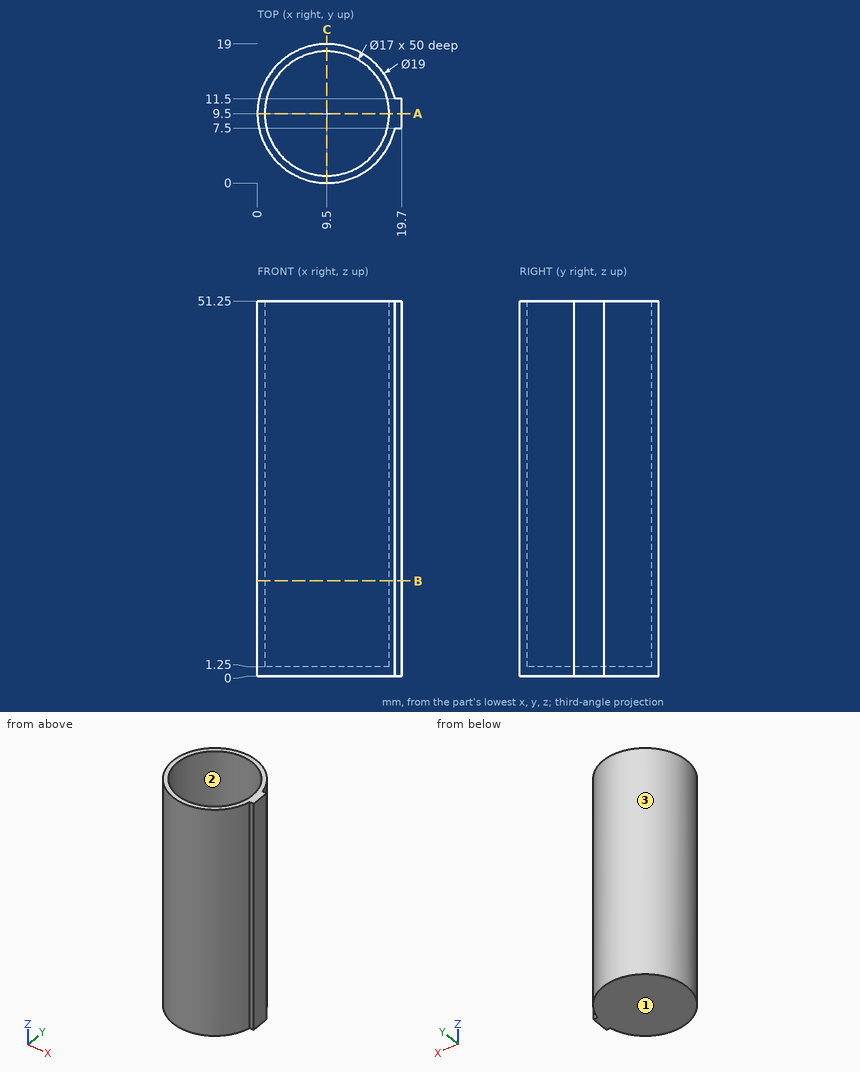
Job drawing, mm, ordinate dimensions from the low corner. One solid piece. Give positions to 0.01 mm unless a question says otherwise; leave off trailing zeros. Write each loop counter-clockwise with the first axis right and the second up, starting at its lowest first coordinate (ties: lowest second). Pieces come first, ordered by that corner, then holes. Notation, with made-up numbers: M 76.25,20 L 86.25,20 A16 cw 86.25,48 Z; hole C -10.75,-39.75 d9. An arc over 180 degrees is marked long. One line per item, written item: value. Start each with the question number.
Q1. Drop flat-ended pins along their axis: pin 1 Ø5 at (x, y) = (8, 12.5) entering from +Z; pin 2 Ø4 at (x, z) = (12.5, 8.5) entering from -Y; pin 3 Ø4 at (y, z) = (16, 6) entering from +X. Give the stop position or say it passes through.
Q2. Saw through at C-C, the plane x = 9.5. Write the cut outline in (y, z).
Q3. Probe probe 1 along Y at (x, z) = (9.5, 36); probe 2 along X at (y, z) = (9.5, 20); probe 3 along Z at (x, y) = (11.5, 11.5). List the from-to ranges inside material, lowest first. Write a range as [from, to].
Q4. Two-plate mould, pull along X, no slides. Class the marked faces 1, 2 and 3: +X half, -X half, draft (parallel to the pull), parting line (faces both ways), or undercut.
Q5. Saw through at A-A, the plane y = 9.5. Write the cut outline in (x, z).
Q6. Saw through at B-B, the plane z = 13. Write the cut outline in (x, y).
Output values:
1. pin 1: stops at z = 1.25
1. pin 2: stops at y = 0.05
1. pin 3: stops at x = 17.87
2. outline: M 0,0 L 19,0 L 19,51.25 L 18,51.25 L 18,1.25 L 1,1.25 L 1,51.25 L 0,51.25 Z
3. probe 1: y = [0, 1], [18, 19]
3. probe 2: x = [0, 1], [18, 19.7]
3. probe 3: z = [0, 1.25]
4. face 1: draft
4. face 2: undercut
4. face 3: parting line
5. outline: M 0,0 L 19.7,0 L 19.7,51.25 L 18,51.25 L 18,1.25 L 1,1.25 L 1,51.25 L 0,51.25 Z
6. outline: M 18.79,7.5 L 19.7,7.5 L 19.7,11.5 L 18.79,11.5 A9.5 ccw long Z; hole C 9.5,9.5 d17
